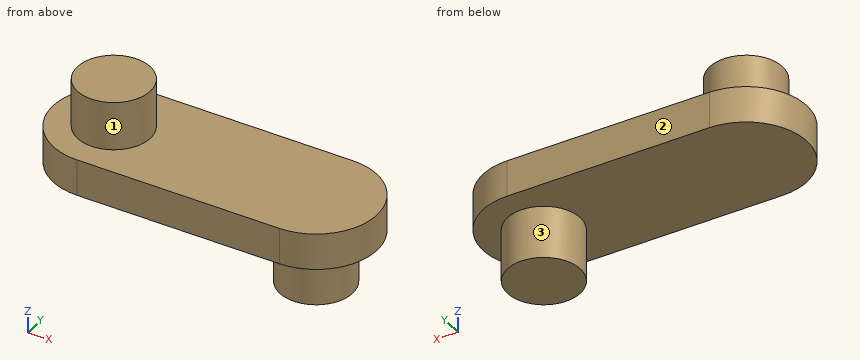
```python
from build123d import *

# Parameters (mm, degrees)
SALIENTE_EXTRUIR1_DEPTH = 9
CROQUIS2_R              = 9
SALIENTE_EXTRUIR2_DEPTH = 12
CROQUIS2_2_R            = 9
SALIENTE_EXTRUIR3_DEPTH = 22


with BuildPart() as part:
    # Croquis1 → Saliente-Extruir1 (new body)
    with BuildSketch(Plane.XY):
        with BuildLine():
            Line((-8.792487614, 13.030881789), (41.207512386, 13.030881789))
            ThreePointArc((41.207512386, 13.030881789), (56.207512386, -1.969118211), (41.207512386, -16.969118211))
            Line((41.207512386, -16.969118211), (-8.792487614, -16.969118211))
            ThreePointArc((-8.792487614, -16.969118211), (-23.792487614, -1.969118211), (-8.792487614, 13.030881789))
        make_face()
    extrude(amount=SALIENTE_EXTRUIR1_DEPTH)

    # Croquis2 → Saliente-Extruir2 (add)
    with BuildSketch(Plane.XY.offset(9)):
        with Locations(Location((-8.792487614, -1.969118211, 0), (0, 0, 180))):
            Circle(CROQUIS2_R)
    extrude(amount=SALIENTE_EXTRUIR2_DEPTH)

    # Croquis2_2 → Saliente-Extruir3 (add)
    with BuildSketch(Plane.XY.offset(9)):
        with Locations((41.207512386, -1.969118211)):
            Circle(CROQUIS2_2_R)
    extrude(amount=-SALIENTE_EXTRUIR3_DEPTH)


solid = part.part
```
CAD build for the part. Positions are in the model's coordinates, mm. Face numbers are marked on the shaded views. A direction names the side the tool comes from. Give positions to 0.01 mm unless a question says otherwise; leave off trailing zeros. Order: outer loops, then holes, each group sorted by start corner. A loop starts at its lowest first (then second) coordinate and runs counter-clockwise, first axis right, second up. Notation, with made-up numbers: M 40,82.5 L 73,82.5 A13 cw 73,94.5 Z; hole C -15.75,39 d3. An arc over 180 degrees is marked long. Put each result on its own line as item: value. Start each with the question number.
(1) Flat gauge pins, fed straight in: pin 1 Ø12 at (x, y) = (24.5, 0.5) entering from -Z; pin 2 Ø1 at (x, z) = (-9.5, 11) entering from +Y. Where does each tip first touch, or does it go through?
(2) Saw through at A-A, the plane y = -6.5. Write the cut outline in (x, z), then the cut area to 3 significant figures.
(3) Which spindle directions (+Z, -Z, +X, -X, +Y, -Y) get a long thin tool onto all of the face, cutting with end or side? Do the marked faces 1, 2 and 3. Say none if no direction does.
(4) Saw through at D-D, the plane y = -1. Write the cut outline in (x, z).
(5) Saw through at B-B, the plane x = 35. Write the cut outline in (y, z), then the cut area to 3 significant figures.
(6) Saw through at C-C, the plane z = 3.5. Write the cut outline in (x, y), then the cut area to 3 significant figures.
(7) Drill centre lines: line 1 along Z through (x, y) = (-10, 7); line 2 along Z through (x, y) = (-10, 3.5); line 3 along X through (y, z) = (4, 8). Where is each one in solid material? Low to high.
Check result:
1. pin 1: stops at z = 0
1. pin 2: stops at y = 7.03
2. outline: M -23.09,0 L 33.43,0 L 33.43,-13 L 48.98,-13 L 48.98,0 L 55.51,0 L 55.51,9 L -1.02,9 L -1.02,21 L -16.57,21 L -16.57,9 L -23.09,9 Z
2. area: 1,100 mm2
3. face 1: +Z
3. face 2: +Z, -Z, +X, -X, +Y
3. face 3: -Z
4. outline: M -23.76,0 L 32.26,0 L 32.26,-13 L 50.16,-13 L 50.16,0 L 56.18,0 L 56.18,9 L 0.16,9 L 0.16,21 L -17.74,21 L -17.74,9 L -23.76,9 Z
5. outline: M -16.97,0 L -8.49,0 L -8.49,-13 L 4.55,-13 L 4.55,0 L 13.03,0 L 13.03,9 L -16.97,9 Z
5. area: 439 mm2
6. outline: M -8.79,-16.97 L 41.21,-16.97 A15 ccw 41.21,13.03 L -8.79,13.03 A15 ccw Z
6. area: 2,210 mm2
7. line 1: z = 0 to 9
7. line 2: z = 0 to 21
7. line 3: x = -22.55 to 54.97
